from build123d import *

# Parameters (mm, degrees)
F0_W     = 76
F0_H     = 36
F1_DEPTH = 1000


# Not quite as in the source:
# - ends of sketch curves that miss each other by under 0.0002 mm in the source are joined


with BuildPart() as f1:
    # F0 (on Front) → F1 (new body)
    with BuildSketch(Plane.XZ):
        with BuildLine():
            ThreePointArc((-37.999999, 20), (-39.4142135624, 19.4142135624), (-40, 17.999999))
            Line((-40, 17.999999), (-40, -18))
            ThreePointArc((-40, -18), (-39.4142128553, -19.4142142695), (-37.999999, -20))
            Line((-37.999999, -20), (38, -20))
            ThreePointArc((38, -20), (39.4142139159, -19.4142132088), (40, -18))
            Line((40, -18), (40, 18))
            ThreePointArc((40, 18), (39.4142139159, 19.4142132088), (38.000001, 20))
            Line((38.000001, 20), (-37.999999, 20))
        make_face()
        Rectangle(F0_W, F0_H, mode=Mode.SUBTRACT)
    extrude(amount=F1_DEPTH)


solid = f1.part
Input: part model. Units: mm. Frame: model coordinates. A direction names the side the tool comes from. Coordinates: 2 decimals unless noted, no trailing zeros. Loops run counter-clockwise (first coordinate to the right, second up) from the corner with the lowest first, then second, coordinate; pieces in that order, holes last. Notation, with made-up numbers: (10, -29.5) -> (16, -29.5) arc R18 cw to (16, 5.5) -> close; hole circle Ø2 at (30.5, 27.25). An arc over 180 degrees is marked (long way). Write each question's results on one line, items separated by ' | '. Start each with the question number.
Q1. Section C-C, the plane y = -300. Return the cut outline in (x, z).
Q2. Section B-B, the plane x = -26. Return the cut outline in (y, z).
Q3. Ray query, line 1 (X direction, y = -748, z = 12.5); line 2 (Z direction, x = 12, y = -334). Return the intervals inside material, ascending. Write a range as from..to.
Q4. Pull-direction query (Z, two-part tool) for faces 1 (the flat face through (-1, -493, -20)), 2 (the flat face through (40, -493, 0)), 3 (the flat face through (-1, -493, 18)); classes: released by +Z, released by -Z, zero draft, split by the parting line, or undercut.
Q5. Reachability of faces 4 (the flat face through (38, -493, 0)), 5 (the flat face through (1, -493, 20)) from +Z, -Z, +X, -X, +Y, -Y: full face, straight path, thin tool, end or side. Return the list, or none.
Q6. Section A-A, the plane z = 2.5. Return the cut outline in (x, y).
Found:
1) outline: (-40, -18) arc R2 ccw to (-38, -20) -> (38, -20) arc R2 ccw to (40, -18) -> (40, 18) arc R2 ccw to (38, 20) -> (-38, 20) arc R2 ccw to (-40, 18) -> close; hole (-38, -18) -> (38, -18) -> (38, 18) -> (-38, 18) -> close
2) outline: (-1000, -20) -> (0, -20) -> (0, -18) -> (-1000, -18) -> close; (-1000, 18) -> (0, 18) -> (0, 20) -> (-1000, 20) -> close
3) line 1: -40..-38, 38..40 | line 2: -20..-18, 18..20
4) face 1: released by -Z | face 2: zero draft | face 3: undercut
5) face 4: +Y, -Y | face 5: +Z, +X, -X, +Y, -Y
6) outline: (-40, -1000) -> (-38, -1000) -> (-38, 0) -> (-40, 0) -> close; (38, -1000) -> (40, -1000) -> (40, 0) -> (38, 0) -> close
